Verification items for the finished model (mm, model axes). A direction names the side the tool comes from. Coordinates: 2 decimals unless noted, no trailing zeros. Loops run counter-clockwise (first coordinate to the right, second up) from the corner with the lowest first, then second, coordinate; pieces in that order, holes last. Notation, with made-up numbers: (16.5, -30.5) - (20.5, -30.5) arc R17 cw to (20.5, -7.5) - close; hole circle Ø4 at (23, 10.5). An arc over 180 degrees is marked (long way). One line per item, written item: value. Start each with the question number.
(1) Section check D-D (y = 4). Record the boundary of the cut face in (x, z) (3 decimals), plus the area to 3 significant figures.
(2) Gauge pin test, flat ends, axial feed: P1, Ø1.9, axis at y = -3.5, z = -15, coming from the -X side; P2, Ø3.5, axis at y = -4, z = -15.5, coming from the +X side; P3, Ø2, axis at y = -2.5, z = 14, coming from the -X side; P4, Ø2.5, axis at y = 14, z = 0, coming from the +X side. Record the tip position at first contact, or that the pin passes through.
(3) Set-up check for faces 1 (the face through (-2.124, 9, 0)), 2 (the face through (-0.75, -3, -13)), 3 (the face through (-7, 0, 0)), 4 (the face through (2.25, -1.9, 16.2)), 5 (the face through (0.75, -3, 13)): record each of +Z, -Z, +X, -X, +Y, -Y from which the full face is reachable in a straight line by a thin tool's end or side.
(4) Thickness scan on probe 1 along Z at (x, y) = (-1.4, -3.5); probe 2 along Z at (x, y) = (1.3, -3.5); probe 3 along X at (y, z) = (-1, -15.5). Record the ranges inside material, lowest first. Write a range as [from, to].
(5) Section check A-A (y = -3.5). Count the separate pieces of the cut face and the enclosed holes in it, plus the area to 3 significant figures.
(6) Section check B-B (z = 0). Record the boundary of the cut face in (x, y) (3 decimals).
(7) Section check C-C (x = 0). Record the boundary of the cut face in (y, z) (3 decimals).
(8) Draft check along X on faces 6 (the face through (9.448, -4.465, -0.197)), 7 (the face through (-1, -3, 18.627)), 8 (the face through (-12.448, -3.451, 0.242)). Enter one of: +X half, -X half, draft (parallel to the pull), parting line (faces both ways), or undercut.
```python
from build123d import *

# Parameters (mm, degrees)
BOSS_EXTRUDE1_DEPTH = 18
SKETCH2_R           = 12.45
SKETCH2_R_2         = 9.45
BOSS_EXTRUDE2_DEPTH = 7
SKETCH3_R           = 12.45
BOSS_EXTRUDE3_DEPTH = 2
CUT_EXTRUDE1_REACH  = 30.085
SKETCH4_R           = 1.45
CUT_EXTRUDE3_REACH  = 32.578
BOSS_EXTRUDE5_START = -7
BOSS_EXTRUDE5_DEPTH = 7
SKETCH8_R           = 1.6
CUT_EXTRUDE4_DEPTH  = 30.783714089
CUT_EXTRUDE5_DEPTH  = 29.739904748


with BuildPart() as part:
    # Sketch1 → Boss-Extrude1 (new body)
    with BuildSketch(Plane(origin=(0, 0, 0), x_dir=(1, 0, 0), z_dir=(0, 1, 0))):
        with BuildLine():
            Line((-5.149418526, 2.325078245), (-5.149418526, -2.325078245))
            ThreePointArc((-5.149418526, -2.325078245), (5.65, 0), (-5.149418526, 2.325078245))
        make_face()
        with BuildLine():
            Line((-2.124418526, 1.541904967), (-2.124418526, -1.541904967))
            ThreePointArc((-2.124418526, -1.541904967), (2.625, 0), (-2.124418526, 1.541904967))
        make_face(mode=Mode.SUBTRACT)
    extrude(amount=BOSS_EXTRUDE1_DEPTH)



with BuildPart() as body_2:
    # Sketch2 → Boss-Extrude2 (new body)
    with BuildSketch(Plane.XZ):
        with Locations(Location((0, 0, 0), (0, 0, 270))):
            Circle(SKETCH2_R)
        with Locations(Location((0, 0, 0), (0, 0, 270))):
            Circle(SKETCH2_R_2, mode=Mode.SUBTRACT)
    extrude(amount=BOSS_EXTRUDE2_DEPTH)


with BuildPart() as part_1:
    add(part.part)

    add(body_2.part)  # Boss-Extrude3 merges body 2
    # Sketch3 → Boss-Extrude3 (add)
    with BuildSketch(Plane.XZ):
        with Locations(Location((0, 0, 0), (0, 0, 270))):
            Circle(SKETCH3_R)
    extrude(amount=BOSS_EXTRUDE3_DEPTH)

    # Sketch4 → Cut-Extrude1 (cut, up to next)
    with BuildSketch(Plane.ZY.offset(5.149418526), mode=Mode.PRIVATE) as cut_extrude1_sk1:
        with Locations((0, 14)):
            Circle(SKETCH4_R)
    cut_extrude1_tool1 = extrude(cut_extrude1_sk1.sketch, amount=-CUT_EXTRUDE1_REACH, mode=Mode.PRIVATE) & part_1.part
    # Sketch4 → Cut-Extrude1 (cut, up to next)
    with BuildSketch(Plane.ZY.offset(5.149418526), mode=Mode.PRIVATE) as cut_extrude1_sk2:
        with Locations((0, 4)):
            Circle(SKETCH4_R)
    cut_extrude1_tool2 = extrude(cut_extrude1_sk2.sketch, amount=-CUT_EXTRUDE1_REACH, mode=Mode.PRIVATE) & part_1.part
    add(cut_extrude1_tool1.solids().sort_by_distance((-5.149419, 14, 0))[0], mode=Mode.SUBTRACT)
    add(cut_extrude1_tool2.solids().sort_by_distance((-5.149419, 4, 0))[0], mode=Mode.SUBTRACT)

    # Sketch6 → Cut-Extrude3 (cut, up to next)
    with BuildSketch(Plane.XZ.offset(7), mode=Mode.PRIVATE) as cut_extrude3_sk1:
        with BuildLine():
            Line((0.75, 9.420191081), (0.75, 12.427389106))
            ThreePointArc((0.75, 12.427389106), (0, 12.45), (-0.75, 12.427389106))
            Line((-0.75, 12.427389106), (-0.75, 9.420191081))
            ThreePointArc((-0.75, 9.420191081), (0, 9.45), (0.75, 9.420191081))
        make_face()
    cut_extrude3_tool1 = extrude(cut_extrude3_sk1.sketch, amount=-CUT_EXTRUDE3_REACH, mode=Mode.PRIVATE) & part_1.part
    # Sketch6 → Cut-Extrude3 (cut, up to next)
    with BuildSketch(Plane.XZ.offset(7), mode=Mode.PRIVATE) as cut_extrude3_sk2:
        with BuildLine():
            Line((0.75, -9.420191081), (0.75, -12.427389106))
            ThreePointArc((0.75, -12.427389106), (0, -12.45), (-0.75, -12.427389106))
            Line((-0.75, -12.427389106), (-0.75, -9.420191081))
            ThreePointArc((-0.75, -9.420191081), (0, -9.45), (0.75, -9.420191081))
        make_face()
    cut_extrude3_tool2 = extrude(cut_extrude3_sk2.sketch, amount=-CUT_EXTRUDE3_REACH, mode=Mode.PRIVATE) & part_1.part
    add(cut_extrude3_tool1.solids().sort_by_distance((0, -7, 10.941262))[0], mode=Mode.SUBTRACT)
    add(cut_extrude3_tool2.solids().sort_by_distance((0, -7, -10.941262))[0], mode=Mode.SUBTRACT)

    # Sketch7 → Boss-Extrude5 (add)
    with BuildSketch(Plane.XZ.offset(7).offset(BOSS_EXTRUDE5_START)):
        with BuildLine():
            Line((-0.75, 12.427389106), (-0.75, 18.627389106))
            Line((-0.75, 18.627389106), (-2.25, 18.627389106))
            Line((-2.25, 18.627389106), (-2.25, 12.244998979))
            ThreePointArc((-2.25, 12.244998979), (-1.502769623, 12.35897178), (-0.75, 12.427389106))
        make_face()
        with BuildLine():
            Line((2.25, 18.627389106), (2.25, 12.244998979))
            ThreePointArc((2.25, 12.244998979), (1.502769623, 12.35897178), (0.75, 12.427389106))
            Line((0.75, 12.427389106), (0.75, 18.627389106))
            Line((0.75, 18.627389106), (2.25, 18.627389106))
        make_face()
        with BuildLine():
            Line((0.75, -12.427389106), (0.75, -18.627389106))
            Line((0.75, -18.627389106), (2.25, -18.627389106))
            Line((2.25, -18.627389106), (2.25, -12.244998979))
            ThreePointArc((2.25, -12.244998979), (1.502769623, -12.35897178), (0.75, -12.427389106))
        make_face()
        with BuildLine():
            Line((-2.25, -18.627389106), (-2.25, -12.244998979))
            ThreePointArc((-2.25, -12.244998979), (-1.502769623, -12.35897178), (-0.75, -12.427389106))
            Line((-0.75, -12.427389106), (-0.75, -18.627389106))
            Line((-0.75, -18.627389106), (-2.25, -18.627389106))
        make_face()
    extrude(amount=BOSS_EXTRUDE5_DEPTH)

    # Sketch8 → Cut-Extrude4 (cut, through all)
    with BuildSketch(Plane.ZY.offset(2.25)):
        with Locations(Location((-15.436194043, -3.5, 0), (0, 0, 180))):
            Circle(SKETCH8_R)
        with Locations(Location((15.436194043, -3.5, 0), (0, 0, 180))):
            Circle(SKETCH8_R)
    extrude(amount=-CUT_EXTRUDE4_DEPTH, mode=Mode.SUBTRACT)

    # Sketch9 → Cut-Extrude5 (cut, through all)
    with BuildSketch(Plane(origin=(0, 0, 0), x_dir=(1, 0, 0), z_dir=(0, 1, 0))):
        with BuildLine():
            Line((-0.75, -9.420191081), (-0.75, -5.6))
            ThreePointArc((-0.75, -5.6), (0, -5.65), (0.75, -5.6))
            Line((0.75, -5.6), (0.75, -9.420191081))
            ThreePointArc((0.75, -9.420191081), (0, -9.45), (-0.75, -9.420191081))
        make_face()
        with BuildLine():
            Line((-0.75, 5.6), (-0.75, 9.420191081))
            ThreePointArc((-0.75, 9.420191081), (0, 9.45), (0.75, 9.420191081))
            Line((0.75, 9.420191081), (0.75, 5.6))
            ThreePointArc((0.75, 5.6), (0, 5.65), (-0.75, 5.6))
        make_face()
    extrude(amount=-CUT_EXTRUDE5_DEPTH, mode=Mode.SUBTRACT)


solid = part_1.part
```
Responses:
1. outline: (-5.149, -2.325) arc R5.65 ccw (long way) to (-5.149, 2.325) - (-5.149, 1.45) - (-2.124, 1.45) - (-2.124, 1.542) arc R2.625 cw (long way) to (-2.124, -1.542) - (-2.124, -1.45) - (-5.149, -1.45) - close
1. area: 69.4 mm²
2. P1: passes through
2. P2: stops at x = 2.25
2. P3: stops at x = -2.25
2. P4: stops at x = 5.65
3. face 1: +Y
3. face 2: -Z, +Y, -Y
3. face 3: -X, +Y
3. face 4: +Z, +X, +Y, -Y
3. face 5: +Z, +Y, -Y
4. probe 1: z = [-18.63, -17.04], [-13.84, -9.35], [9.35, 13.84], [17.04, 18.63]
4. probe 2: z = [-18.63, -17.04], [-13.84, -9.36], [9.36, 13.84], [17.04, 18.63]
4. probe 3: x = [-2.25, -0.75], [0.75, 2.25]
5. separate pieces: 6
5. enclosed holes: 0
5. area: 216 mm²
6. outline: (-12.45, -7) - (-9.45, -7) - (-9.45, -2) - (9.45, -2) - (9.45, -7) - (12.45, -7) - (12.45, 0) - (5.65, 0) - (5.65, 18) - (2.625, 18) - (2.625, 0) - (-2.124, 0) - (-2.124, 2.55) - (-5.149, 2.55) - (-5.149, 0) - (-12.45, 0) - close; (-5.149, 5.45) - (-2.124, 5.45) - (-2.124, 12.55) - (-5.149, 12.55) - close; (-5.149, 15.45) - (-2.124, 15.45) - (-2.124, 18) - (-5.149, 18) - close
7. outline: (-2, -5.65) - (18, -5.65) - (18, -2.625) - (0, -2.625) - (0, 2.625) - (18, 2.625) - (18, 5.65) - (-2, 5.65) - close
8. face 6: undercut
8. face 7: draft
8. face 8: -X half
